Source: three-view drawing plus pictorial views. Frame: mm from the lowest corner of the part. A direction names the side the tool comes from. Give positions to 0.01 mm unless a question says otherwise; leave off trailing zeros. Loops run counter-clockwise (first coordinate to the right, second up) from the corner with the lowest first, then second, coordinate; pieces in that order, holes last. Notation, with made-up numbers: M 30.25,-29.75 L 46.25,-29.75 A27 ccw 46.25,4.25 Z; hole C -9.5,89 d5. An arc over 180 degrees is marked long. Answer as a JSON object with one key per item and string values. Group by question number.
1) Access query for the marked faces 1 and 2. Directions: +Z, -Z, +X, -X, +Y, -Y. A direction counts if a zero-diameter tool reaches every point of the face in a straight line with its end or side. Return the directions, or none.
2) Section query A-A on x = 4. Return loops of the section in (y, z), plus the area to 3 significant figures.
3) Section query B-B on y = 0.2. Return loops of the section in (x, z).
4) Ray query, L1, parallel to Z at x = 4.75, y = 0.1; L2, parallel to X at y = 0.85, z = 2.5; L3, parallel to X at y = 0.3, z = 2. Return the intervals inside material, ascending.
5) Draft query along X for the marked faces 3, 4, 5 and 6. Return one class per face: +X half, -X half, draft (parallel to the pull), parting line (faces both ways), or undercut.
6) Section query C-C on z = 3.5. Return loops of the section in (x, y), plus the area to 3 significant figures.
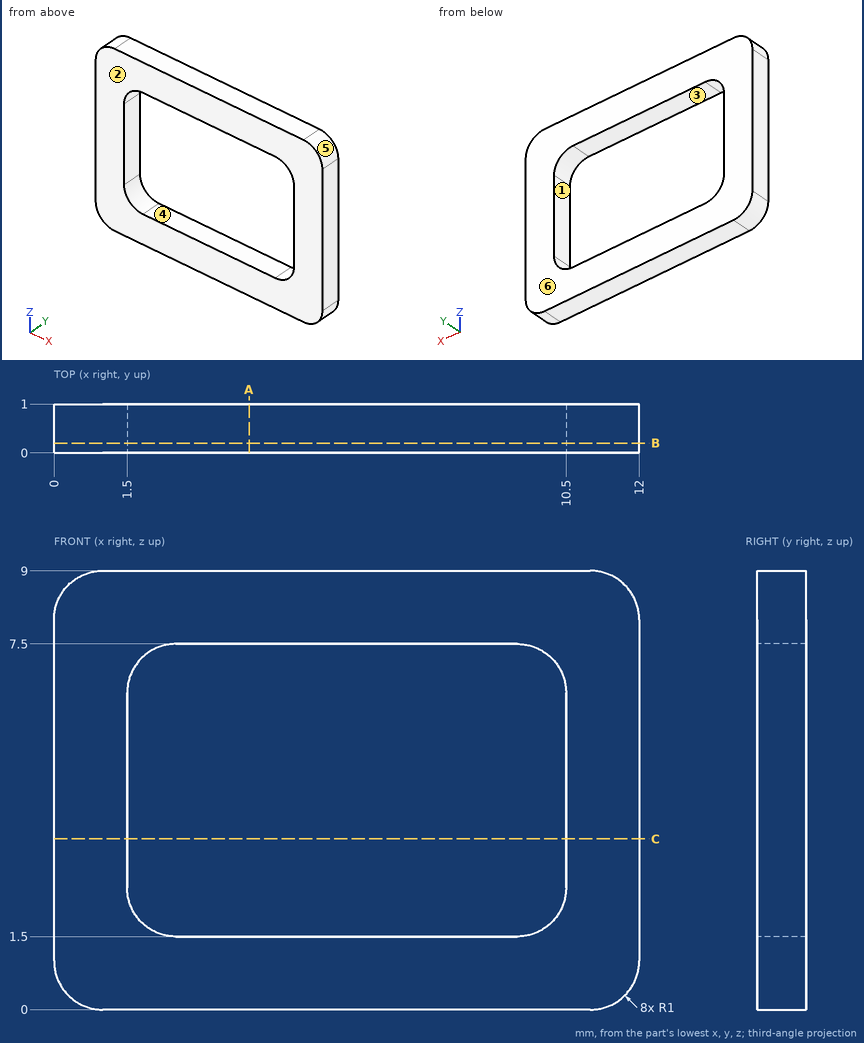
Output:
{
 "1": {"face 1": "+Y, -Y", "face 2": "+Z, -Z, +X, -X, -Y"},
 "2": {"outline": "M 0,0 L 1,0 L 1,1.5 L 0,1.5 Z; M 0,7.5 L 1,7.5 L 1,9 L 0,9 Z", "area": "3.00 mm^2"},
 "3": {"outline": "M 0,1 A1 ccw 1,0 L 11,0 A1 ccw 12,1 L 12,8 A1 ccw 11,9 L 1,9 A1 ccw 0,8 Z; hole M 1.5,2.5 A1 ccw 2.5,1.5 L 9.5,1.5 A1 ccw 10.5,2.5 L 10.5,6.5 A1 ccw 9.5,7.5 L 2.5,7.5 A1 ccw 1.5,6.5 Z"},
 "4": {"L1": "z = 0 to 1.5, 7.5 to 9", "L2": "x = 0 to 1.5, 10.5 to 12", "L3": "x = 0 to 1.63, 10.37 to 12"},
 "5": {"face 3": "undercut", "face 4": "undercut", "face 5": "+X half", "face 6": "draft"},
 "6": {"outline": "M 0,0 L 1.5,0 L 1.5,1 L 0,1 Z; M 10.5,0 L 12,0 L 12,1 L 10.5,1 Z", "area": "3.00 mm^2"}
}
